The model under review builds one solid part; all positions refer to its coordinate system, in mm. A direction names the side the tool comes from. Give positions to 0.01 mm unless a question says otherwise; leave off trailing zeros. Write each loop counter-clockwise with the first axis right and the second up, starting at its lowest first coordinate (ties: lowest second). Pieces come first, ordered by that corner, then holes.
from build123d import *

# Parameters (mm, degrees)
F0_W      = 9
F0_H      = 10.6
F1_DEPTH  = 9
F3_DEPTH  = 1
F4_R      = 2.95
F5_DEPTH  = 4
F6_R      = 0.5
F7_DEPTH  = 0.3
F8_R      = 0.5
F9_DEPTH  = 0.3
F10_R     = 1.8
F11_DEPTH = 10


with BuildPart() as f1:
    # F0 (on Top) → F1 (new body)
    with BuildSketch(Plane.XY):
        Rectangle(F0_W, F0_H)
    extrude(amount=F1_DEPTH)

    # F2 (on face) → F3 (join)
    with BuildSketch(Plane(origin=(-4.5, 0, 0), x_dir=(0, -1, 0), z_dir=(-1, 0, 0))):
        with BuildLine():
            Line((3, 2.3542486889), (3, 7.6457513111))
            ThreePointArc((3, 7.6457513111), (0, 9), (-3, 7.6457513111))
            Line((-3, 7.6457513111), (-3, 2.3542486889))
            ThreePointArc((-3, 2.3542486889), (0, 1), (3, 2.3542486889))
        make_face()
    extrude(amount=F3_DEPTH)

    # F4 (on face) → F5 (join)
    with BuildSketch(Plane(origin=(-5.5, 0, 0), x_dir=(0, -1, 0), z_dir=(-1, 0, 0))):
        with Locations((0, 5)):
            Circle(F4_R)
    extrude(amount=F5_DEPTH)

    # F6 (on face) → F7 (join)
    with BuildSketch(Plane(origin=(0, 5.3, 0), x_dir=(-1, 0, 0), z_dir=(0, 1, 0))):
        with BuildLine():
            Line((-4.5, 5.4), (-4.5, 6.5))
            Line((-4.5, 6.5), (-6.8220781011, 6.5))
            ThreePointArc((-6.8220781011, 6.5), (-9.3, 5.95), (-6.8220781011, 5.4))
            Line((-6.8220781011, 5.4), (-4.5, 5.4))
        make_face()
        with Locations((-8, 5.95)):
            Circle(F6_R, mode=Mode.SUBTRACT)
    extrude(amount=-F7_DEPTH)

    # F8 (on face) → F9 (join)
    with BuildSketch(Plane.XZ.offset(5.3)):
        with BuildLine():
            Line((4.5, 6.5), (4.5, 5.4))
            Line((4.5, 5.4), (6.8220781011, 5.4))
            ThreePointArc((6.8220781011, 5.4), (9.3, 5.95), (6.8220781011, 6.5))
            Line((6.8220781011, 6.5), (4.5, 6.5))
        make_face()
        with Locations((8, 5.95)):
            Circle(F8_R, mode=Mode.SUBTRACT)
    extrude(amount=-F9_DEPTH)

    # F10 (on face) → F11 (cut)
    with BuildSketch(Plane(origin=(-9.5, 0, 0), x_dir=(0, -1, 0), z_dir=(-1, 0, 0))):
        with Locations((0, 5)):
            Circle(F10_R)
    extrude(amount=-F11_DEPTH, mode=Mode.SUBTRACT)


solid = f1.part
1) Tool access review of faces 1 (the cylindrical face through (-4.57, 0.39, 3.243)), 2 (the flat face through (7, 5, 6)), 3 (the flat face through (-5, 3, 5)), 4 (the flat face through (-5, -3, 5)), 5 (the cylindrical face through (-5, 0, 1)): name each direction out of +Z, -Z, +X, -X, +Y, -Y from which nothing blocks a thin tool from reaching the whole face with its end or side.
2) Consider section A-A, the plane x = 8. Give the boundary of the cut face in (y, z), then the cut area to 3 significant figures.
3) To check wall thickness, follow probe 1 along Z at (x, y) = (8, 5.15); probe 2 along Y at (x, z) = (-1, 6.5); probe 3 along X at (y, z) = (4, 5.75). State the ranges of each line that lie inside material, in increasing order.
4) Consider section C-C, the plane x = -8.25. Give the boundary of the cut face in (y, z).
5) Consider section B-B, the plane z = 5. Give the boundary of the cut face in (x, y), then the cut area to 3 significant figures.
6) Insertion check: pin 1 (1.8 mm diameter, centred on y = 0.5, z = 5.5, fed in from -X); pin 2 (1.5 mm diameter, centred on y = 2, z = 1.5, fed in from -X). Each pin has a flat end and moves straight along its axis. Give the tip position at first contact, or say it passes through.
7) The part is to be moulded in two halves that separate along Z. For faces 6 (the cylindrical face through (7.73, 5.15, 6.37)), 7 (the cylindrical face through (-7.472, 0.384, 7.925)), 8 (the flat face through (-4.5, -2, 1)), say which applies: +Z half, -Z half, draft (parallel to the pull), parting line (faces both ways), or undercut.
Answer block:
1. face 1: -X
1. face 2: +Z, -Z, +X
1. face 3: +Z, -Z, -X, +Y
1. face 4: +Z, -Z, -X, -Y
1. face 5: -Z, -X
2. outline: (-5.3, 4.65) - (-5, 4.65) - (-5, 5.45) - (-5.3, 5.45) - close; (-5.3, 6.45) - (-5, 6.45) - (-5, 7.25) - (-5.3, 7.25) - close; (5, 4.65) - (5.3, 4.65) - (5.3, 5.45) - (5, 5.45) - close; (5, 6.45) - (5.3, 6.45) - (5.3, 7.25) - (5, 7.25) - close
2. area: 0.960 mm2
3. probe 1: z = 4.65 to 5.45, 6.45 to 7.25
3. probe 2: y = -5.3 to -0.99, 0.99 to 5.3
3. probe 3: x = -4.5 to 4.5
4. outline: circle Ø5.9 at (0, 5); hole circle Ø3.6 at (0, 5)
5. outline: (-9.5, -2.95) - (-5.5, -2.95) - (-5.5, -3) - (-4.5, -3) - (-4.5, -5.3) - (4.5, -5.3) - (4.5, 5.3) - (-4.5, 5.3) - (-4.5, 3) - (-5.5, 3) - (-5.5, 2.95) - (-9.5, 2.95) - (-9.5, 1.8) - (0.5, 1.8) - (0.5, -1.8) - (-9.5, -1.8) - close; (7.11, -5.3) - (8.89, -5.3) - (8.89, -5) - (7.11, -5) - close; (7.11, 5) - (8.89, 5) - (8.89, 5.3) - (7.11, 5.3) - close
5. area: 90.1 mm2
6. pin 1: stops at x = 0.5
6. pin 2: stops at x = -5.5
7. face 6: undercut
7. face 7: parting line
7. face 8: draft
